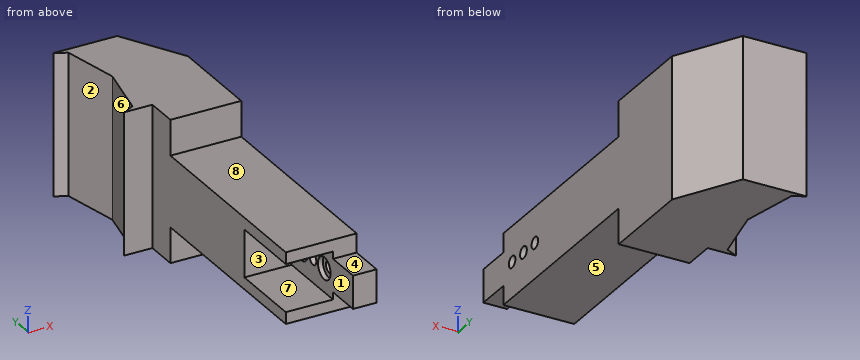
Autodesk Inventor part; units mm, degrees
ref_plane "Work Plane1" through (0, 0, -15) normal (0, 0, 1) x (1, 0, 0)
ref_plane "YZ Plane" through (0, 0, 0) normal (1, 0, 0) x (0, 1, 0)
ref_plane "XZ Plane" through (0, 0, 0) normal (0, 1, 0) x (-1, 0, 0)
sketch "Sketch1" plane through (0, 0, 0) normal (0, 0, 1) x (1, 0, 0)
  line L0 (0, 0) -> (25, 0)
  line L1 (25, 0) -> (25, 40)
  line L2 (25, 40) -> (0, 40)
  line L3 (0, 40) -> (0, 0)
  dimension "d1" = 25
  dimension "d2" = 40
  dimension "d3" = 25
extrude "Extrusion1" add sketch "Sketch1" against normal blind 30
sketch "Sketch2" plane through (25, 0, 0) normal (1, 0, 0) x (0, 0, -1)
  line L0 (0, 0) -> (30, 0)
  circle A0 centre (15, 6.56) radius 2.46
extrude "Extrusion2" cut sketch "Sketch2" against normal blind 30
sketch "Sketch3" plane through (0, 0, 0) normal (-1, 0, 0) x (0, 0, 1)
  line L0 (0, 0) -> (-30, 0)
  line L1 (-25.05, 0) -> (-4.95, 0)
  line L2 (-4.95, 0) -> (-4.95, 33.12)
  line L3 (-4.95, 33.12) -> (-25.05, 33.12)
  line L4 (-25.05, 33.12) -> (-25.05, 0)
  dimension "d11" = 20.1
extrude "Extrusion3" cut sketch "Sketch3" against normal blind 20
sketch "Sketch4" plane through (0, 0, 0) normal (0, -1, 0) x (1, 0, 0)
  line L0 (20, -4.95) -> (20, -25.05)
  line L1 (20, -15) -> (25, -15)
  line L2 (25, 0) -> (25, -30)
  line L3 (20, -8.025) -> (25, -8.025)
  line L4 (25, -8.025) -> (25, -21.975)
  line L5 (25, -21.975) -> (20, -21.975)
  line L6 (20, -21.975) -> (20, -8.025)
  line L7 (20, -8.025) -> (25, -21.975) construction
  line L8 (25, -8.025) -> (20, -21.975) construction
  line L9 (25, -12.54) -> (25, -17.46)
  point P0 (0, 0)
  point P1 (22.5, -15)
  dimension "d14" = 13.95
extrude "Extrusion4" add sketch "Sketch4" along normal blind 15
sketch "Sketch5" plane through (20, 0, 0) normal (-1, 0, 0) x (0, 0, 1)
  circle A0 centre (-15, 6.56) radius 2.46
  circle A1 centre (-15, 6.56) radius 4.7025
  circle A2 centre (-15, 6.56) radius 2.46
  circle A3 centre (-15, 6.56) radius 2.46
  point P0 (0, 0)
  dimension "d17" = 9.405
extrude "Extrusion5" cut sketch "Sketch5" against normal blind 2.1
sketch "Sketch6" plane through (25, 0, 0) normal (1, 0, 0) x (0, 0, -1)
  circle A0 centre (15, 6.56) radius 4.7025
  line L0 (15, 6.56) -> (15, 23.56)
  circle A1 centre (15, 23.56) radius 2.46
  point P0 (0, 0)
  dimension "d20" = 17
  dimension "d21" = 4.92
extrude "Extrusion6" cut sketch "Sketch6" against normal blind 10 contours A1
sketch "Sketch7" plane through (20, 0, 0) normal (-1, 0, 0) x (0, 0, 1)
  circle A0 centre (-15, 23.56) radius 2.46
  circle A1 centre (-15, 23.56) radius 4.7025
  point P0 (0, 0)
  dimension "d24" = 9.405
extrude "Extrusion7" cut sketch "Sketch7" against normal blind 2.1
sketch "Sketch9" plane through (25, 0, 0) normal (1, 0, 0) x (0, 0, -1)
  circle A0 centre (15, 6.56) radius 2.46
  circle A1 centre (15, 6.56) radius 2.46
  circle A2 centre (15, 23.56) radius 2.46
  circle A3 centre (15, 23.56) radius 2.46
  line L0 (30, 40) -> (30, 0)
  line L1 (30, 0) -> (30, 40)
  line L2 (30, 40) -> (0, 40)
  line L3 (0, 40) -> (0, 0)
  line L4 (0, 0) -> (8.025, 0)
  line L5 (21.975, 0) -> (21.975, -15)
  line L6 (21.975, -15) -> (8.025, -15)
  line L7 (8.025, -15) -> (8.025, 0)
  line L8 (0, 0) -> (8.025, 0)
  line L9 (21.975, 0) -> (30, 0)
extrude "Extrusion8" add sketch "Sketch9" along normal blind 5
sketch "Sketch10" plane through (0, 40, 0) normal (0, 1, 0) x (1, 0, 0)
  line L0 (0, 30) -> (30, 30)
  line L1 (30, 0) -> (0, 0)
  line L2 (0, 30) -> (30, 30)
  line L3 (30, 30) -> (30, 0)
  line L4 (30, 0) -> (0, 0)
  line L5 (0, 0) -> (0, 30)
extrude "Extrusion9" add sketch "Sketch10" along normal blind 30
sketch "Sketch12" plane through (30, 0, 0) normal (1, 0, 0) x (0, 0, -1)
  circle A0 centre (15, 6.56) radius 2.46
  line L0 (15, 6.56) -> (15, 15.06)
  circle A1 centre (15, 15.06) radius 2.525
  point P0 (0, 0)
  dimension "d31" = 8.5
  dimension "d33" = 5.05
extrude "Extrusion10" cut sketch "Sketch12" against normal blind 30 contours A1
sketch "Sketch14" plane through (0, 0, 0) normal (0, 0, 1) x (1, 0, 0)
  line L0 (30, 70) -> (0, 70)
  line L1 (0, 70) -> (0, 85)
  line L2 (30, 0) -> (30, 70)
  line L3 (30, 122.5) -> (30, 70)
  line L4 (30, 105) -> (30, 100)
  line L5 (-12, 153) -> (15, 153)
  line L6 (-7, 150.5) -> (-12, 153)
  line L7 (-7, 102.5) -> (-12, 100)
  line L8 (-7, 102.5) -> (-2, 126.5)
  line L9 (-2, 126.5) -> (-7, 150.5)
  line L10 (30, 126.5) -> (15, 153)
  line L11 (30, 122.5) -> (30, 126.5)
  line L12 (0, 85) -> (0, 100)
  line L13 (0, 100) -> (-12, 100)
  point P0 (0, 0)
  dimension "d90" = 12
extrude "Extrusion12" add sketch "Sketch14" against normal blind 30
sketch "Sketch15" plane through (0, 0, -25.05) normal (-1, 0, 0) x (0, 0, 1)
  line L0 (0, 33.12) -> (20.1, 33.12)
  line L1 (20.1, 33.12) -> (20.1, 0)
  line L2 (0, 33.12) -> (20.1, 33.12)
  line L3 (20.1, 33.12) -> (20.1, 31.1)
  line L4 (20.1, 31.1) -> (0, 31.1)
  line L5 (0, 31.1) -> (0, 33.12)
  point P0 (25.05, 0)
  dimension "d57" = 2.02
extrude "Extrusion13" add sketch "Sketch15" against normal blind 20
sketch "Sketch25" plane through (0, 0, 0) normal (0, 0, 1) x (1, 0, 0)
  line L0 (0, 100) -> (-12, 100)
  line L1 (0, 100) -> (-12, 100)
  line L2 (-12, 100) -> (-7, 102.5)
  line L3 (-12, 100) -> (-7, 102.5)
  line L4 (-7, 102.5) -> (-2, 126.5)
  line L5 (-7, 102.5) -> (-2, 126.5)
  line L6 (-2, 126.5) -> (-7, 150.5)
  line L7 (-2, 126.5) -> (-7, 150.5)
  line L8 (-7, 150.5) -> (-12, 153)
  line L9 (-7, 150.5) -> (-12, 153)
  line L10 (-12, 153) -> (15, 153)
  line L11 (-12, 153) -> (15, 153)
  line L12 (15, 153) -> (30, 126.5)
  line L13 (15, 153) -> (30, 126.5)
  line L14 (30, 126.5) -> (30, 86.5)
  line L15 (30, 0) -> (30, 126.5)
  line L16 (30, 86.5) -> (0, 86.5)
  line L17 (0, 100) -> (0, 0)
  line L18 (0, 86.5) -> (0, 100)
  dimension "d91" = 40
  dimension "d92" = 30
extrude "Extrusion14" add sketch "Sketch25" along normal blind 15
ref_plane "Work Plane1" through (0, 0, -15) normal (0, 0, 1) x (1, 0, 0)
mirror "Mirror1" about plane through (0, 0, -15) normal (0, 0, 1) of "Extrusion14"
properties part number "rec_b_48mm_x_60mm"
Design review of the part built by this model. Coordinates are the model's own, in mm. Face numbers are marked on the shaded views. A direction names the side the tool comes from. Coordinates: 2 decimals unless noted, no trailing zeros. Order: outer loops, then holes, each group sorted by start corner. A loop starts at its lowest first (then second) coordinate and runs counter-clockwise, first axis right, second up.
Item 1: Take a section at D-D, the plane z = 11.5. Write out the cut boundary in (x, y).
Item 2: Take a section at B-B, the plane y = 15.06. Write out the cut boundary in (x, z) (3 decimals).
Item 3: For line 1 (Z direction, x = 25, y = 6.56); line 2 (Y direction, x = 20.95, z = -15) (1 decimal); line 3 (Y direction, x = 26.25, z = -15) (3 decimals), list the stretches that pass through material, from the lowest coordinate up.
Item 4: Take a section at A-A, the plane z = -15. Count the separate pieces of the cut face and the enclosed holes in it, then the cut area to 3 significant figures.
Item 5: Take a section at C-C, the plane x = 27. Write out the cut boundary in (y, z) (3 decimals).
Item 6: For pin 1 Ø12 at (y, z) = (82.5, 7) entering from +X; pin 2 Ø6.5 at (y, z) = (15.06, -15) entering from -X; pin 3 Ø11 at (x, y) = (22.5, -8.5) entering from +Z (3 decimals); pin 4 Ø1 at (x, z) = (24, 7.5) entering from -Y, all flat-tipped, find the tip position at first contact; note any pin that passes through.
Item 7: For the marked faces 5, 6, 7 and 8, list the 3-axis set-ups (+Z, -Z, +X, -X, +Y, -Y) from which the entire face can be reached by the end or side of a thin tool; tool diameter is ignored.
Item 8: The part is to be moulded in two halves that separate along Z. For the marked faces 1, 2, 3 and 4, say which applies: pulls with the +Z half, pulls with the -Z half, needs draft (parallel to the pull), parting line crosses it, or undercut.
The answers:
1. outline: (-12, 100) - (0, 100) - (0, 86.5) - (30, 86.5) - (30, 126.5) - (15, 153) - (-12, 153) - (-7, 150.5) - (-2, 126.5) - (-7, 102.5) - close
2. outline: (0, -30) - (30, -30) - (30, -17.525) - (20, -17.525) - (20, -25.05) - (0, -25.05) - close; (0, -4.95) - (20, -4.95) - (20, -12.475) - (30, -12.475) - (30, 0) - (0, 0) - close
3. line 1: z = -30 to -17.46, -12.54 to 0
3. line 2: y = -15 to 1.9, 11.3 to 12.5, 17.6 to 18.9, 28.3 to 142.5
3. line 3: y = -15 to 4.1, 9.02 to 12.535, 17.585 to 21.1, 26.02 to 133.125
4. separate pieces: 4
4. enclosed holes: 0
4. area: 4,020 mm2
5. outline: (-15, -21.975) - (0, -21.975) - (0, -30) - (86.5, -30) - (86.5, -45) - (131.8, -45) - (131.8, 15) - (86.5, 15) - (86.5, 0) - (0, 0) - (0, -8.025) - (-15, -8.025) - close; hole circle Ø4.92 at (6.56, -15); hole circle Ø5.05 at (15.06, -15); hole circle Ø4.92 at (23.56, -15)
6. pin 1: stops at x = 30
6. pin 2: stops at x = 20
6. pin 3: stops at z = -8.025
6. pin 4: stops at y = 86.5
7. face 5: -Z, +X, -X, -Y
7. face 6: +Z, -Z, -X
7. face 7: -X, -Y
7. face 8: +Z, +X, -X, -Y
8. face 1: undercut
8. face 2: needs draft
8. face 3: undercut
8. face 4: pulls with the +Z half
